from build123d import *

# Parameters (mm, degrees)
SKETCH1_R           = 12.5
SKETCH1_R_2         = 4
BOSS_EXTRUDE1_DEPTH = 12
SKETCH3_W           = 48.002845368
SKETCH3_H           = 76.2
CUT_EXTRUDE5_DEPTH  = 13
BOSS_EXTRUDE3_DEPTH = 3


with BuildPart() as part:
    # Sketch1 → Boss-Extrude1 (new body)
    with BuildSketch(Plane(origin=(0, 0, 0), x_dir=(1, 0, 0), z_dir=(0, 1, 0))):
        with BuildLine():
            Line((67.27241336, 38.839745962), (129.903810568, 75))
            ThreePointArc((129.903810568, 75), (150, 0), (129.903810568, -75))
            Line((129.903810568, -75), (67.27241336, -38.839745962))
            ThreePointArc((67.27241336, -38.839745962), (64.860603811, -37.840741737), (62.27241336, -37.5))
            Line((62.27241336, -37.5), (-25.048094716, -37.5))
            ThreePointArc((-25.048094716, -37.5), (-32.119162528, -34.571067812), (-35.048094716, -27.5))
            Line((-35.048094716, -27.5), (-35.048094716, 27.5))
            ThreePointArc((-35.048094716, 27.5), (-32.119162528, 34.571067812), (-25.048094716, 37.5))
            Line((-25.048094716, 37.5), (62.27241336, 37.5))
            ThreePointArc((62.27241336, 37.5), (64.860603811, 37.840741737), (67.27241336, 38.839745962))
        make_face()
        Circle(SKETCH1_R, mode=Mode.SUBTRACT)
        with Locations((30, 0)):
            Circle(SKETCH1_R_2, mode=Mode.SUBTRACT)
        with Locations((-21.213203436, 21.213203436)):
            Circle(SKETCH1_R_2, mode=Mode.SUBTRACT)
        with Locations((-21.213203436, -21.213203436)):
            Circle(SKETCH1_R_2, mode=Mode.SUBTRACT)
    extrude(amount=BOSS_EXTRUDE1_DEPTH)

    # Sketch3 → Cut-Extrude5 (cut, through all)
    with BuildSketch(Plane(origin=(0, 12, 0), x_dir=(1, 0, 0), z_dir=(0, 1, 0))):
        with Locations((131.301422684, 0)):
            Rectangle(SKETCH3_W, SKETCH3_H)
    extrude(amount=-CUT_EXTRUDE5_DEPTH, mode=Mode.SUBTRACT)

    # Sketch4 → Boss-Extrude3 (add)
    with BuildSketch(Plane(origin=(0, 12, 0), x_dir=(1, 0, 0), z_dir=(0, 1, 0))):
        Polygon((107.3, -38.1), (107.3, 0), (102.3, 0), (102.3, -43.1), (107.3, -43.1), (132.7, -43.1), (132.7, -38.1), align=None)
        Polygon((107.3, 0), (107.3, 38.1), (132.7, 38.1), (132.7, 43.1), (107.3, 43.1), (102.3, 43.1), (102.3, 0), align=None)
    extrude(amount=BOSS_EXTRUDE3_DEPTH)


solid = part.part
Read the model definition and answer for the solid it produces. Units are mm, in the model's axes. A direction names the side the tool comes from. Round coordinates to 2 decimals unless told otherwise and drop trailing zeros. Write each loop counter-clockwise with the first axis right and the second up, starting at its lowest first coordinate (ties: lowest second). Pieces come first, ordered by that corner, then holes. Notation, with made-up numbers: (2, -16.5) - (58, -16.5) arc R25 ccw to (58, 17.5) - close; hole circle Ø8 at (-20.75, -38). An arc over 180 degrees is marked (long way). One line per question, with ' | ' between items. Start each with the question number.
1. Section B-B (x = -10) is taken. Determine the outline of the cut face in (y, z).
2. Section C-C (y = 6.25) is taken. Determine the outline of the cut face in (x, z), and give its area (3 significant figures).
3. For faces 5 (the face through (107.3, 7, 1)), 6 (the face through (18, 6, -37.5)), 7 (the face through (-35.048, 6, 0)), determine the directions among +Z, -Z, +X, -X, +Y, -Y from which every point of the face is accessible in a straight line to the end or side of a thin tool.
4. For a pull along X with two mould halves and no side action, classify faces 1 (the face through (19, 6, 37.5)), 2 (the face through (138.618, 5.916, -57.316)), 3 (the face through (-24.16, 5.92, 18.51)), 4 (the face through (-32.2, 5.92, -34.49)) as +X half, -X half, draft (parallel to the pull), parting line (faces both ways), or undercut.
5. Find the intervals of material crossed by probe 1 along X at (y, z) = (7.5, 0); probe 2 along X at (y, z) = (4.5, 3.5); probe 3 along Z at (x, y) = (58.5, 0.75), in increasing order. Write a range as [from, to].
6. Each of these flat-tipped pins is pushed along its axis until it touches: pin 1 (3.5 mm diameter, centred on x = 123.5, y = 13.5, fed in from +Z); pin 2 (1.5 mm diameter, centred on y = 14, z = 39.5, fed in from +X); pin 3 (3 mm diameter, centred on x = 107, y = 3, fed in from -Z). Where does it stop, or does it pass through?
7. Section A-A (z = 0) is taken. Determine the outline of the cut face in (x, y), and give its area (3 significant figures).
8. Section D-D (x = 30) is taken. Determine the outline of the cut face in (y, z).
Filled in:
1) outline: (0, -37.5) - (12, -37.5) - (12, -7.5) - (0, -7.5) - close; (0, 7.5) - (12, 7.5) - (12, 37.5) - (0, 37.5) - close
2) outline: (-35.05, -27.5) arc R10 ccw to (-25.05, -37.5) - (62.27, -37.5) arc R10 cw to (67.27, -38.84) - (129.9, -75) arc R150 ccw to (145.08, -38.1) - (107.3, -38.1) - (107.3, 38.1) - (145.08, 38.1) arc R150 ccw to (129.9, 75) - (67.27, 38.84) arc R10 cw to (62.27, 37.5) - (-25.05, 37.5) arc R10 ccw to (-35.05, 27.5) - close; hole circle Ø8 at (-21.21, -21.21); hole circle Ø8 at (-21.21, 21.21); hole circle Ø25 at (0, 0); hole circle Ø8 at (30, 0) | area: 13,000 mm²
3) face 5: +X, +Y, -Y | face 6: -Z, -X, +Y, -Y | face 7: +Z, -Z, -X, +Y, -Y
4) face 1: draft | face 2: +X half | face 3: undercut | face 4: -X half
5) probe 1: [-35.05, -12.5], [12.5, 26], [34, 107.3] | probe 2: [-35.05, -12], [12, 28.06], [31.94, 107.3] | probe 3: [-37.5, 37.5]
6) pin 1: z = 71.82 | pin 2: x = 132.7 | pin 3: z = -62.64
7) outline: (-35.05, 0) - (-12.5, 0) - (-12.5, 12) - (-35.05, 12) - close; (12.5, 0) - (26, 0) - (26, 12) - (12.5, 12) - close; (34, 0) - (107.3, 0) - (107.3, 15) - (102.3, 15) - (102.3, 12) - (34, 12) - close | area: 1,330 mm²
8) outline: (0, -37.5) - (12, -37.5) - (12, -4) - (0, -4) - close; (0, 4) - (12, 4) - (12, 37.5) - (0, 37.5) - close
